For this review, take the finished solid that the model builds, in its own axes (mm). Give positions to 0.01 mm unless a question says otherwise; leave off trailing zeros. Write each loop counter-clockwise with the first axis right and the second up, starting at its lowest first coordinate (ties: lowest second). Pieces come first, ordered by that corner, then holes.
Q1. We need section C-C (z = -34). Give the number of separate pieces and of enclosed holes in the cut face, then the cut area to 3 significant figures.
Q2. We need section B-B (y = -3.5). Write out the cut boundary in (x, z).
Q3. Mouldability with a two-part tool opening along X and no side actions: class faces 1 (the flat face through (-1, -6.35, 13)), 2 (the cylindrical face through (2.013, -2.379, 90.514)), 3 (the cylindrical face through (77.38, -2.38, -47)), 4 (the cylindrical face through (-15.51, -3.13, 46.28)) as released by +X, released by -X, zero draft, split by the parting line, or undercut.
Q4. We need section A-A (x = 0). Write out the cut boundary in (y, z).
Q5. For line 1 (Z direction, x = 3, y = -1); line 2 (Z direction, x = 0, y = -5); line 3 (X direction, y = -5.75, z = -16.5), list the stretches that pass through material, from the lowest coordinate up.
Q6. Insertion check: P1, Ø1.5, axis at x = 31.5, y = -2.5, coming from the -Z side. The pin has a flat end and moves straight along its axis. Give the tip position at first contact, or say it passes through.
```python
from build123d import *

# Parameters (mm, degrees)
F0_R         = 19.5450228134
F0_R_2       = 12.3084359059
F1_DEPTH     = 6.35
F2_T4_ANGLE  = 186.4329686672
F2_S5_R      = 36.413303104
F2_T6_DEPTH  = 41
F2_S7_R      = 34.3943026377
F2_T8_DEPTH  = 41
F2_T12_ANGLE = 186.4329686672
F2_S13_R     = 36.413303104
F2_T14_DEPTH = 44
F2_S15_R     = 34.3943026377
F2_T16_DEPTH = 44
F2_T20_ANGLE = 186.4329686672
F2_S21_R     = 36.413303104
F2_T22_DEPTH = 43
F2_S23_R     = 34.3943026377
F2_T24_DEPTH = 43


# Not quite as in the source:
# - a fillet or chamfer that OpenCascade refuses, or shapes differently, is made with other operations: its cross-section is extruded or revolved along the edge and cut away or added


with BuildPart() as f1:
    # F0 (on Front) → F1 (new body)
    with BuildSketch(Plane.XZ):
        with BuildLine():
            ThreePointArc((45.7058369334, 33.6726559303), (41.6121725533, 47.6126804082), (32.3941794324, 58.8425946254))
            ThreePointArc((32.3941794324, 58.8425946254), (1.3289124245, 90.5489995431), (-32.2304944376, 61.495374328))
            ThreePointArc((-32.2304944376, 61.495374328), (-49.0277697558, 45.6463332306), (-52.0142939153, 22.7460879204))
            ThreePointArc((-52.0142939153, 22.7460879204), (-62.0398770524, 12.2308583337), (-67.1562714864, -1.3671149894))
            ThreePointArc((-67.1562714864, -1.3671149894), (-79.0821901038, -44.1236278525), (-37.1413091645, -58.6601141235))
            ThreePointArc((-37.1413091645, -58.6601141235), (-15.0169992894, -65.2824607147), (6.3084569819, -56.4187438507))
            ThreePointArc((6.3084569819, -56.4187438507), (20.4277044991, -59.8435387419), (34.7620920539, -57.4754796359))
            ThreePointArc((34.7620920539, -57.4754796359), (77.7532776793, -46.4253716906), (69.3718036021, -2.8352602045))
            ThreePointArc((69.3718036021, -2.8352602045), (64.0447690452, 19.6361274841), (45.7058369334, 33.6726559303))
        make_face()
        with Locations((-50.3812096523, -29.0876049548)):
            Circle(F0_R, mode=Mode.SUBTRACT)
        with Locations((50.3812096523, -29.0876049548)):
            Circle(F0_R, mode=Mode.SUBTRACT)
        Circle(F0_R_2, mode=Mode.SUBTRACT)
        with Locations((0, 58.1752099097)):
            Circle(F0_R, mode=Mode.SUBTRACT)
    extrude(amount=F1_DEPTH)

    # F2: fillet of radius 1.524 on 3 edges, made by hand


with BuildPart() as f2_tool2:
    # F2_s3 → F2_t4 (revolve)
    with BuildSketch(Plane(origin=(5.6170399672, 0, 57.627710491), x_dir=(0, 1, 0), z_dir=(-0.0970114178, 0, -0.9952832686))):
        with BuildLine():
            ThreePointArc((-4.826, 26.7573938379), (-5.9036307345, 26.3110245724), (-6.35, 25.2333938379))
            Line((-6.35, 25.2333938379), (-6.35, 26.7573938379))
            Line((-6.35, 26.7573938379), (-4.826, 26.7573938379))
        make_face()
    revolve(axis=Axis((0, -6.35, 58.1752099097), (0, -1, 0)), revolution_arc=F2_T4_ANGLE)

    # F2_s5 → F2_t6 (cut, symmetric)
    with BuildSketch(Plane.XZ.offset(5.6)):
        with Locations((9.423343912, 30.5889336513)):
            Circle(F2_S5_R)
    extrude(amount=F2_T6_DEPTH, both=True, mode=Mode.SUBTRACT)

    # F2_s7 → F2_t8 (cut, symmetric)
    with BuildSketch(Plane.XZ.offset(5.6)):
        with Locations((-18.3950397685, 30.0065152183)):
            Circle(F2_S7_R)
    extrude(amount=F2_T8_DEPTH, both=True, mode=Mode.SUBTRACT)


with BuildPart() as f1_1:
    add(f1.part)

    # F2_t1: cut F2_tool2
    add(f2_tool2.part, mode=Mode.SUBTRACT)


with BuildPart() as f2_tool10:
    # F2_s11 → F2_t12 (revolve)
    with BuildSketch(Plane(origin=(47.0985412635, 0, -33.6783545512), x_dir=(0, 1, 0), z_dir=(-0.8134348857, 0, 0.5816559866))):
        with BuildLine():
            ThreePointArc((-4.826, 26.7573938379), (-5.9036307345, 26.3110245724), (-6.35, 25.2333938379))
            Line((-6.35, 25.2333938379), (-6.35, 26.7573938379))
            Line((-6.35, 26.7573938379), (-4.826, 26.7573938379))
        make_face()
    revolve(axis=Axis((50.3812096523, -6.35, -29.0876049548), (0, -1, 0)), revolution_arc=F2_T12_ANGLE)

    # F2_s13 → F2_t14 (cut, symmetric)
    with BuildSketch(Plane.XZ.offset(5.6)):
        with Locations((21.7791216607, -23.4553220421)):
            Circle(F2_S13_R)
    extrude(amount=F2_T14_DEPTH, both=True, mode=Mode.SUBTRACT)

    # F2_s15 → F2_t16 (cut, symmetric)
    with BuildSketch(Plane.XZ.offset(5.6)):
        with Locations((35.1839243423, 0.927314134)):
            Circle(F2_S15_R)
    extrude(amount=F2_T16_DEPTH, both=True, mode=Mode.SUBTRACT)


with BuildPart() as f1_2:
    add(f1_1.part)

    # F2_t9: cut F2_tool10
    add(f2_tool10.part, mode=Mode.SUBTRACT)


with BuildPart() as f2_tool18:
    # F2_s19 → F2_t20 (revolve)
    with BuildSketch(Plane(origin=(-52.7155812308, 0, -23.9493559398), x_dir=(0, 1, 0), z_dir=(0.9104463035, 0, 0.4136272821))):
        with BuildLine():
            ThreePointArc((-4.826, 26.7573938379), (-5.9036307345, 26.3110245724), (-6.35, 25.2333938379))
            Line((-6.35, 25.2333938379), (-6.35, 26.7573938379))
            Line((-6.35, 26.7573938379), (-4.826, 26.7573938379))
        make_face()
    revolve(axis=Axis((-50.3812096523, -6.35, -29.0876049548), (0, -1, 0)), revolution_arc=F2_T20_ANGLE)

    # F2_s21 → F2_t22 (cut, symmetric)
    with BuildSketch(Plane.XZ.offset(5.6)):
        with Locations((-31.2024655727, -7.1336116092)):
            Circle(F2_S21_R)
    extrude(amount=F2_T22_DEPTH, both=True, mode=Mode.SUBTRACT)

    # F2_s23 → F2_t24 (cut, symmetric)
    with BuildSketch(Plane.XZ.offset(5.6)):
        with Locations((-16.7888845738, -30.9338293523)):
            Circle(F2_S23_R)
    extrude(amount=F2_T24_DEPTH, both=True, mode=Mode.SUBTRACT)


with BuildPart() as f1_3:
    add(f1_2.part)

    # F2_t17: cut F2_tool18
    add(f2_tool18.part, mode=Mode.SUBTRACT)


solid = f1_3.part
```
Computed:
1. separate pieces: 3
1. enclosed holes: 0
1. area: 565 mm2
2. outline: (-67.16, -1.37) arc R32.4 ccw to (-37.14, -58.66) arc R34.39 ccw to (6.31, -56.42) arc R36.41 ccw to (34.76, -57.48) arc R32.4 ccw to (69.37, -2.84) arc R34.39 ccw to (45.71, 33.67) arc R36.41 ccw to (32.39, 58.84) arc R32.4 ccw to (-32.23, 61.5) arc R34.39 ccw to (-52.01, 22.75) arc R36.41 ccw to start; hole circle Ø39.09 at (-50.38, -29.09); hole circle Ø39.09 at (0, 58.18); hole circle Ø24.62 at (0, 0); hole circle Ø39.09 at (50.38, -29.09)
3. face 1: zero draft
3. face 2: split by the parting line
3. face 3: undercut
3. face 4: undercut
4. outline: (-6.35, -60.95) - (0, -60.95) - (0, -12.31) - (-6.35, -12.31) - close; (-6.35, 12.31) - (0, 12.31) - (0, 38.63) - (-6.35, 38.63) - close; (-6.35, 77.72) - (0, 77.72) - (0, 90.58) - (-4.83, 90.58) arc R1.52 ccw to (-6.35, 89.05) - close
5. line 1: z = -59.07 to -11.94, 11.94 to 38.86, 77.49 to 90.44
5. line 2: z = -60.95 to -12.31, 12.31 to 38.63, 77.72 to 90.57
5. line 3: x = -79.9 to -65.33, -35.43 to 35.43, 65.33 to 79.9
6. P1: stops at z = -58.75
